Verification items for the finished model (mm, model axes). A direction names the side the tool comes from. Give positions to 0.01 mm unless a question says otherwise; leave off trailing zeros. Write each loop counter-clockwise with the first axis right and the second up, starting at its lowest first coordinate (ties: lowest second). Pieces come first, ordered by that corner, then holes. Notation, with made-up numbers: (-24, 8.5) -> (-1, 8.5) arc R16 cw to (-1, 26.5) -> close; hole circle Ø5 at (25, 71). An arc over 180 degrees is marked (long way). Answer as CSV lines item,"result". Start each with the question number.
1) Gauge pin test, flat ends, axial feed: pin 1 Ø3 at (y, z) = (-9.5, 1.5) entering from +X; pin 2 Ø1.2 at (x, z) = (66.5, 2) entering from -Y; pin 3 Ø7 at (x, y) = (62.2, 7.5) entering from -Z; pin 4 Ø4 at (x, y) = (62, 9) entering from +Z. Record the tip position at first contact, or that the pin passes through.
2) Mould release check, pull along X, two halves, no side actions. Record for faces 5 (the cylindrical face through (65.895, 5.968, 2.521)), 6 (the flat face through (59, 7, 1)), 7 (the flat face through (44, -25, 2)), 8 (the flat face through (18, 0, 2)): released by +X, released by -X, zero draft, split by the parting line, or undercut.
3) Material ranges on L1, parallel to X at y = 4, z = 3.5; L2, parallel to X at y = 7.5, z = 0.05; L3, parallel to Z at x = 39, y = -11.5, recorded low to high.
4) Tool access check on faces 1 (the flat face through (77.2, 7, 6)), 2 (the flat face through (40, -50, 2)), 3 (the flat face through (21, 8, 1)), 4 (the flat face through (62, 0, 2)). Record the directions out of +Z, -Z, +X, -X, +Y, -Y that give a thin tool (end or side, any length) a straight path to the whole face; none if there is none.
5) Sectioned sample at A-A on z = 5.25. Record the cut outline in (x, y).
6) Sectioned sample at D-D on y = -32.5. Record the cut outline in (x, z).
7) Sectioned sample at C-C on y = 7.5. Give the number of separate pieces and of enclosed holes in the cut face, and give its area (3 significant figures).
```python
from build123d import *

# Parameters (mm, degrees)
SKETCH1_W           = 80
SKETCH1_H           = 15
BOSS_EXTRUDE1_DEPTH = 4
SKETCH2_W           = 2.8
SKETCH2_H           = 15
BOSS_EXTRUDE2_DEPTH = 5
SKETCH3_W           = 1.2
SKETCH3_H           = 6
BOSS_EXTRUDE3_DEPTH = 0.4
SKETCH4_W           = 1.2
SKETCH4_H           = 6
BOSS_EXTRUDE4_DEPTH = 0.4
FILLET1_R           = 0.4
FILLET2_R           = 3
SKETCH5_W           = 8
SKETCH5_H           = 50
BOSS_EXTRUDE5_DEPTH = 4
FILLET3_R           = 3
SKETCH6_R           = 4
CUT_EXTRUDE1_DEPTH  = 3
SKETCH7_R           = 2
CUT_EXTRUDE2_DEPTH  = 3
CHAMFER1_SIZE       = 1


with BuildPart() as part:
    # Sketch1 → Boss-Extrude1 (new body)
    with BuildSketch(Plane.XY):
        with Locations((40, 7.5)):
            Rectangle(SKETCH1_W, SKETCH1_H)
    extrude(amount=BOSS_EXTRUDE1_DEPTH)

    # Sketch2 → Boss-Extrude2 (add)
    with BuildSketch(Plane.XY.offset(4)):
        with Locations((1.4, 7.5)):
            Rectangle(SKETCH2_W, SKETCH2_H)
        with Locations((78.6, 7.5)):
            Rectangle(SKETCH2_W, SKETCH2_H)
    extrude(amount=BOSS_EXTRUDE2_DEPTH)

    # Sketch3 → Boss-Extrude3 (add)
    with BuildSketch(Plane(origin=(2.8, 0, 0), x_dir=(0, 0, -1), z_dir=(1, 0, 0))):
        with Locations((-7.6, 7.5)):
            Rectangle(SKETCH3_W, SKETCH3_H)
    extrude(amount=BOSS_EXTRUDE3_DEPTH)

    # Sketch4 → Boss-Extrude4 (add)
    with BuildSketch(Plane.ZY.offset(-77.2)):
        with Locations((7.6, 7.5)):
            Rectangle(SKETCH4_W, SKETCH4_H)
    extrude(amount=BOSS_EXTRUDE4_DEPTH)

    # Fillet1
    fillet1_edges = [part.edges().sort_by_distance(p)[0] for p in [
        (3.2, 10.5, 7.6),
        (3.2, 4.5, 7.6),
        (76.8, 10.5, 7.6),
        (76.8, 4.5, 7.6),
        (76.8, 7.5, 8.2),
        (3.2, 7.5, 8.2),
    ]]
    fillet(fillet1_edges, radius=FILLET1_R - 0.0001)  # a hair under: the kernel refuses the full size

    # Fillet2
    fillet2_edges = [part.edges().sort_by_distance(p)[0] for p in [
        (80, 0, 4.5),
        (80, 15, 4.5),
        (0, 0, 4.5),
        (0, 15, 4.5),
    ]]
    fillet(fillet2_edges, radius=FILLET2_R)

    # Sketch5 → Boss-Extrude5 (add)
    with BuildSketch(Plane.XY):
        with Locations((40, -25)):
            Rectangle(SKETCH5_W, SKETCH5_H)
    extrude(amount=BOSS_EXTRUDE5_DEPTH)

    # Fillet3
    fillet3_edges = [part.edges().sort_by_distance(p)[0] for p in [
        (36, 0, 2),
        (36, -50, 2),
        (44, -50, 2),
        (44, 0, 2),
    ]]
    fillet(fillet3_edges, radius=FILLET3_R)

    # Sketch6 → Cut-Extrude1 (cut)
    with BuildSketch(Plane.XY.offset(4)):
        with Locations((17.8, 7.5)):
            Circle(SKETCH6_R)
        with Locations((62.2, 7.5)):
            Circle(SKETCH6_R)
    extrude(amount=-CUT_EXTRUDE1_DEPTH, mode=Mode.SUBTRACT)

    # Sketch7 → Cut-Extrude2 (cut)
    with BuildSketch(Plane.XY.offset(1)):
        with Locations((17.8, 7.5)):
            Circle(SKETCH7_R)
        with Locations((62.2, 7.5)):
            Circle(SKETCH7_R)
    extrude(amount=-CUT_EXTRUDE2_DEPTH, mode=Mode.SUBTRACT)

    # Chamfer1
    chamfer1_edges = [part.edges().sort_by_distance(p)[0] for p in [
        (15.8, 7.5, 1),
        (60.2, 7.5, 1),
    ]]
    chamfer(chamfer1_edges, length=CHAMFER1_SIZE - 0.0001)  # a hair under: the kernel refuses the full size


solid = part.part
```
Ans:
1,pin 1,"stops at x = 44"
1,pin 2,"stops at y = 0"
1,pin 3,"stops at z = 0"
1,pin 4,"stops at z = 1"
2,face 5,"undercut"
2,face 6,"undercut"
2,face 7,"released by +X"
2,face 8,"zero draft"
3,L1,"x = 0 to 15.86, 19.74 to 60.26, 64.14 to 80"
3,L2,"x = 0 to 15.75, 19.85 to 60.15, 64.25 to 80"
3,L3,"z = 0 to 4"
4,face 1,"none"
4,face 2,"+Z, -Z, +X, -X, -Y"
4,face 3,"+Z"
4,face 4,"+Z, -Z, +X, -Y"
5,outline,"(0, 3) arc R3 ccw to (2.8, 0.01) -> (2.8, 14.99) arc R3 ccw to (0, 12) -> close; (77.2, 0.01) arc R3 ccw to (80, 3) -> (80, 12) arc R3 ccw to (77.2, 14.99) -> close"
6,outline,"(36, 0) -> (44, 0) -> (44, 4) -> (36, 4) -> close"
7,separate pieces,"3"
7,enclosed holes,"0"
7,area,"291 mm²"
